```python
from build123d import *

# Parameters (mm, degrees)
SKETCH_W        = 130
SKETCH_H        = 32
PAD_DEPTH       = 4
SKETCH001_R     = 2.35
SKETCH001_R_2   = 2.75
POCKET_DEPTH    = 4.001
SKETCH002_R     = 2.25
POCKET001_DEPTH = 4.001
CHAMFER_SIZE    = 2
FILLET_R        = 5


with BuildPart() as part:
    # Sketch → Pad (new body)
    with BuildSketch(Plane.XY):
        Rectangle(SKETCH_W, SKETCH_H)
    extrude(amount=PAD_DEPTH)

    # Sketch001 → Pocket (cut, through all)
    with BuildSketch(Plane.XY.offset(4)):
        with Locations((-35, 9)):
            Circle(SKETCH001_R)
        with Locations((-58.997728, -9)):
            Circle(SKETCH001_R)
        with Locations((-59, 9)):
            Circle(SKETCH001_R)
        with Locations((35, 9)):
            Circle(SKETCH001_R)
        with Locations((59, -9)):
            Circle(SKETCH001_R)
        with Locations((59, 9)):
            Circle(SKETCH001_R)
        with Locations((-47, 9)):
            Circle(SKETCH001_R_2)
        with Locations((-47, -11)):
            Circle(SKETCH001_R_2)
        with Locations((47, 9)):
            Circle(SKETCH001_R_2)
        with Locations((47, -11)):
            Circle(SKETCH001_R_2)
        with Locations((-21, 0)):
            Circle(SKETCH001_R_2)
        with Locations((21, 0)):
            Circle(SKETCH001_R_2)
        with Locations((-35, -9)):
            Circle(SKETCH001_R)
        with Locations((35, -9)):
            Circle(SKETCH001_R)
    extrude(amount=-POCKET_DEPTH, mode=Mode.SUBTRACT)

    # Sketch002 → Pocket001 (cut, through all)
    with BuildSketch(Plane.XY.offset(4)):
        with Locations((-10, 10)):
            Circle(SKETCH002_R)
        with Locations((-10, 0)):
            Circle(SKETCH002_R)
        with Locations((10, 10)):
            Circle(SKETCH002_R)
        with Locations((10, 0)):
            Circle(SKETCH002_R)
        with Locations((0, 10)):
            Circle(SKETCH002_R)
        Circle(SKETCH002_R)
        with Locations((0, -10)):
            Circle(SKETCH002_R)
        with Locations((-10, -10)):
            Circle(SKETCH002_R)
        with Locations((10, -10)):
            Circle(SKETCH002_R)
        with Locations((-20, 10)):
            Circle(SKETCH002_R)
        with Locations((20, 10)):
            Circle(SKETCH002_R)
        with Locations((20, -10)):
            Circle(SKETCH002_R)
        with Locations((-20, -10)):
            Circle(SKETCH002_R)
    extrude(amount=-POCKET001_DEPTH, mode=Mode.SUBTRACT)

    # Chamfer
    chamfer_edges = [part.edges().sort_by_distance(p)[0] for p in [
        (0, 16, 4),
    ]]
    chamfer(chamfer_edges, length=CHAMFER_SIZE)

    # Fillet
    fillet_edges = [part.edges().sort_by_distance(p)[0] for p in [
        (-65, 16, 1),
        (65, 16, 1),
        (-65, -16, 2),
        (65, -16, 2),
    ]]
    fillet(fillet_edges, radius=FILLET_R)


solid = part.part
```
Can you work these out from the model? Positions are in its coordinate system, mm. Coordinates: 2 decimals unless noted, no trailing zeros. Order: outer loops, then holes, each group sorted by start corner. A loop starts at its lowest first (then second) coordinate and runs counter-clockwise, first axis right, second up.
1. If we section it at D-D (x = 21): Please give me the cut outline in (y, z), then the cut area to 3 significant figures.
2. I need wall thicknesses on line 1 (Y direction, x = 35, z = 1.85); line 2 (Y direction, x = -20.5, z = 3.55); line 3 (Y direction, x = -20, z = 0.45). Which ranges of each line are inside material? Lowest first, please.
3. If we section it at C-C (x = -10): Please give me the cut outline in (y, z), then the cut area to 3 significant figures.
4. If we section it at A-A (y = 0): Please give me the cut outline in (x, z).
5. Thinking about a two-plate mould opening in Y: for faces 1 (the face through (-11.66, -8.48, 2.03)), 2 (the face through (65, 0, 2)), 3 (the face through (64, 14, 2)), which applies, +Y half, -Y half, draft (parallel to the pull), parting line (faces both ways), or undercut?
6. If we section it at B-B (x = -47): Please give me the cut outline in (y, z).
Entries:
1. outline: (-16, 0) - (-12.02, 0) - (-12.02, 4) - (-16, 4) - close; (-7.98, 0) - (-2.75, 0) - (-2.75, 4) - (-7.98, 4) - close; (2.75, 0) - (7.98, 0) - (7.98, 4) - (2.75, 4) - close; (12.02, 0) - (16, 0) - (16, 2) - (14, 4) - (12.02, 4) - close
1. area: 71.8 mm2
2. line 1: y = -16 to -11.35, -6.65 to 6.65, 11.35 to 16
2. line 2: y = -16 to -12.19, -7.81 to -2.7, 2.7 to 7.81, 12.19 to 14.45
2. line 3: y = -16 to -12.25, -7.75 to -2.56, 2.56 to 7.75, 12.25 to 16
3. outline: (-16, 0) - (-12.25, 0) - (-12.25, 4) - (-16, 4) - close; (-7.75, 0) - (-2.25, 0) - (-2.25, 4) - (-7.75, 4) - close; (2.25, 0) - (7.75, 0) - (7.75, 4) - (2.25, 4) - close; (12.25, 0) - (16, 0) - (16, 2) - (14, 4) - (12.25, 4) - close
3. area: 72.0 mm2
4. outline: (-65, 0) - (-23.75, 0) - (-23.75, 4) - (-65, 4) - close; (-18.25, 0) - (-12.25, 0) - (-12.25, 4) - (-18.25, 4) - close; (-7.75, 0) - (-2.25, 0) - (-2.25, 4) - (-7.75, 4) - close; (2.25, 0) - (7.75, 0) - (7.75, 4) - (2.25, 4) - close; (12.25, 0) - (18.25, 0) - (18.25, 4) - (12.25, 4) - close; (23.75, 0) - (65, 0) - (65, 4) - (23.75, 4) - close
5. face 1: undercut
5. face 2: draft
5. face 3: +Y half
6. outline: (-16, 0) - (-13.75, 0) - (-13.75, 4) - (-16, 4) - close; (-8.25, 0) - (6.25, 0) - (6.25, 4) - (-8.25, 4) - close; (11.75, 0) - (16, 0) - (16, 2) - (14, 4) - (11.75, 4) - close
